Part print with two shaded views. Sizes in mm from the minimum x, y, z corner. A direction names the side the tool comes from. Give positions to 0.01 mm unless a question says otherwise; leave off trailing zeros. Write each loop counter-clockwise with the first axis right and the second up, starting at its lowest first coordinate (ties: lowest second). Pieces come first, ordered by that corner, then holes. Notation, with made-up numbers: (64, -40) -> (86, -40) arc R14 cw to (86, -28) -> close; hole circle Ø5 at (12, -1.75). An arc over 180 degrees is marked (long way). Answer in a Markdown table with one row per item. Add a question column.
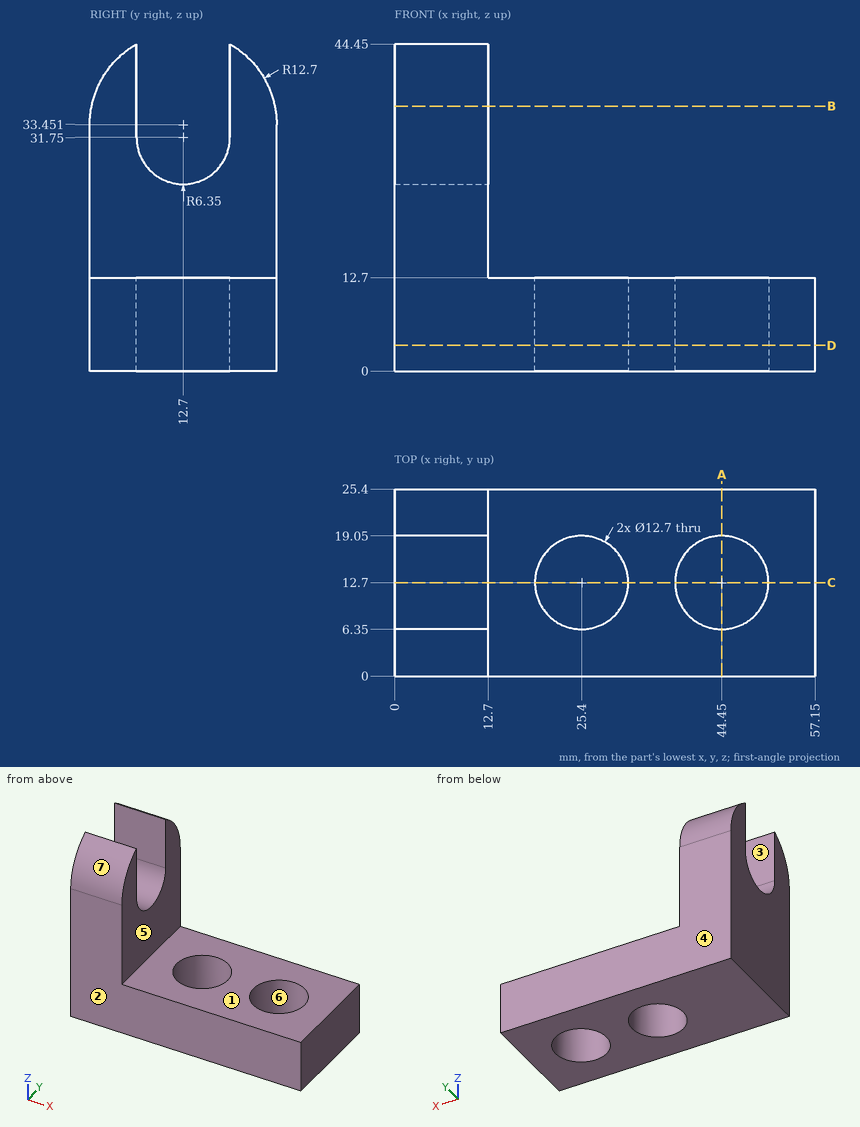
Item 1: Slice it at D-D, the plane z = 3.5. List the corners of the cut face in (x, y).
Item 2: Slice it at C-C, the plane y = 12.7. List the corners of the cut face in (x, z).
Item 3: Drop flat-ended pins along their axis: pin 1 Ø8 at (y, z) = (16.5, 33) entering from +X; pin 2 Ø7.5 at (x, y) = (38, 10) entering from +Z. Give the stop position or say it passes through.
Item 4: Probe L1, parallel to Y at x = 25.4, z = 9.5; L2, parallel to X at y = 9.25, z = 11; L3, parallel to Z at x = 33, y = 22.5. List the from-to ranges inside material, lowest first. Write a range as from..to.
Item 5: Slice it at B-B, the plane z = 36. List the corners of the cut face in (x, y).
Item 6: Slice it at A-A, the plane x = 44.45. List the corners of the cut face in (y, z), then the cut area to 3 significant figures.
Item 7: Which spindle directions (+Z, -Z, +X, -X, +Y, -Y) get a long thin tool onto all of the face, cutting with end or side? Do the marked faces 1, 2 and 3. Say none if no direction does.
Item 8: Mould opens along Y. For the marked faces 4, 5, 6 and 7 say: released by +Y, released by -Y, zero draft, split by the parting line, or undercut.
Answer key:
| question | item | result |
|---|---|---|
| 1 | outline | (0, 0) -> (57.15, 0) -> (57.15, 25.4) -> (0, 25.4) -> close; hole circle Ø12.7 at (25.4, 12.7); hole circle Ø12.7 at (44.45, 12.7) |
| 2 | outline | (0, 0) -> (19.05, 0) -> (19.05, 12.7) -> (12.7, 12.7) -> (12.7, 25.4) -> (0, 25.4) -> close; (31.75, 0) -> (38.1, 0) -> (38.1, 12.7) -> (31.75, 12.7) -> close; (50.8, 0) -> (57.15, 0) -> (57.15, 12.7) -> (50.8, 12.7) -> close |
| 3 | pin 1 | stops at x = 12.7 |
| 3 | pin 2 | stops at z = 12.7 |
| 4 | L1 | y = 0..6.35, 19.05..25.4 |
| 4 | L2 | x = 0..20.07, 30.73..39.12, 49.78..57.15 |
| 4 | L3 | z = 0..12.7 |
| 5 | outline | (0, 0.26) -> (12.7, 0.26) -> (12.7, 6.35) -> (0, 6.35) -> close; (0, 19.05) -> (12.7, 19.05) -> (12.7, 25.14) -> (0, 25.14) -> close |
| 6 | outline | (0, 0) -> (6.35, 0) -> (6.35, 12.7) -> (0, 12.7) -> close; (19.05, 0) -> (25.4, 0) -> (25.4, 12.7) -> (19.05, 12.7) -> close |
| 6 | area | 161 mm² |
| 7 | face 1 | +Z, +X, +Y, -Y |
| 7 | face 2 | +Z, -Z, +X, -X, -Y |
| 7 | face 3 | +Z, +X, -X |
| 8 | face 4 | released by +Y |
| 8 | face 5 | zero draft |
| 8 | face 6 | undercut |
| 8 | face 7 | released by -Y |
